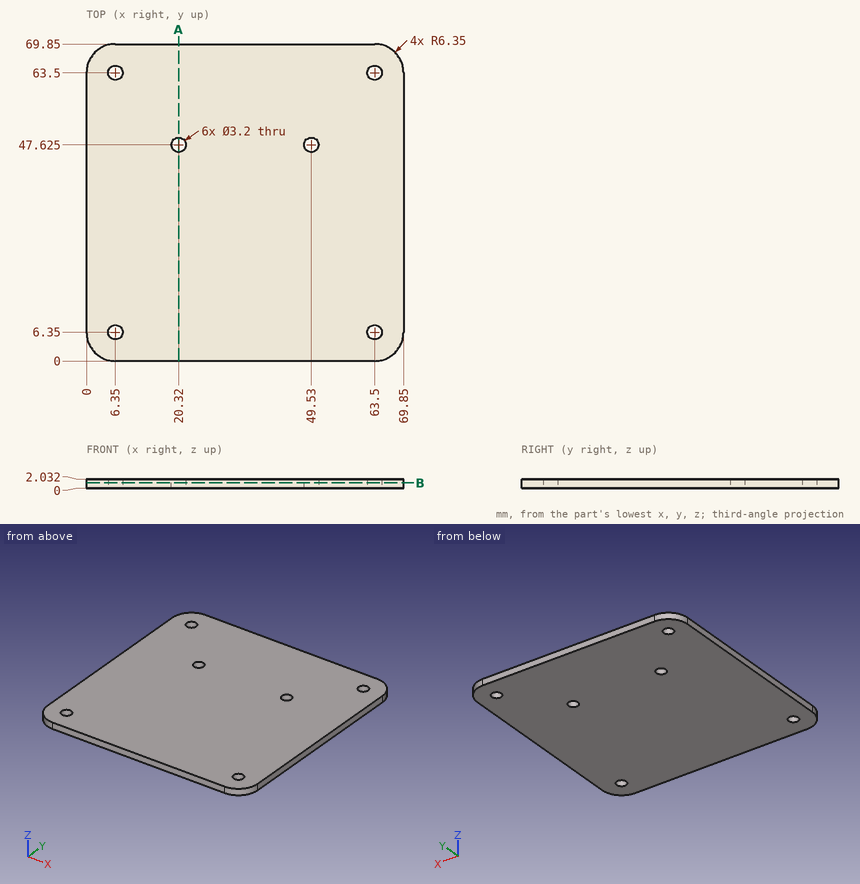
Design review of the part shown in the three views and the two pictorial views. Dimensions are in mm from the part's minimum x, y and z. Give positions to 0.01 mm unless a question says otherwise; leave off trailing zeros. Write each loop counter-clockwise with the first axis right and the second up, starting at its lowest first coordinate (ties: lowest second). Pieces come first, ordered by that corner, then holes. Notation, with made-up numbers: M 14,42 L 26,42 A22 cw 26,73 Z; hole C 23.25,-10.5 d2. An arc over 180 degrees is marked long. One line per item, written item: value.
1) For P1, Ø4, axis at x = 49.53, y = 47.625, coming from the -Z side; P2, Ø2.5, axis at x = 63.5, y = 6.35, coming from the -Z side, all flat-tipped, find the tip position at first contact; note any pin that passes through.
Results are:
P1: stops at z = 0
P2: passes through
2) For line 1 (X direction, y = 63.5, z = 0.7); line 2 (Y direction, x = 64, z = 1.6), list the stretches that pass through material, from the lowest coordinate up. Write a range as from..to.
Results are:
line 1: x = 0..4.75, 7.95..61.9, 65.1..69.85
line 2: y = 0.02..4.83, 7.87..61.98, 65.02..69.83
3) Take a section at B-B, the plane z = 1.2. Write out the cut boundary in (x, y) (3 decimals).
Results are:
outline: M 0,6.35 A6.35 ccw 6.35,0 L 63.5,0 A6.35 ccw 69.85,6.35 L 69.85,63.5 A6.35 ccw 63.5,69.85 L 6.35,69.85 A6.35 ccw 0,63.5 Z; hole C 6.35,6.35 d3.2; hole C 6.35,63.5 d3.2; hole C 20.32,47.625 d3.2; hole C 49.53,47.625 d3.2; hole C 63.5,6.35 d3.2; hole C 63.5,63.5 d3.2
4) Take a section at A-A, the plane x = 20.32. Write out the cut boundary in (y, z) (3 decimals), then the cut area to 3 significant figures.
Results are:
outline: M 0,0 L 46.025,0 L 46.025,2.032 L 0,2.032 Z; M 49.225,0 L 69.85,0 L 69.85,2.032 L 49.225,2.032 Z
area: 135 mm²
